Autodesk Inventor part; units mm, degrees
ref_plane "YZ Plane" through (0, 0, 0) normal (1, 0, 0) x (0, 1, 0)
ref_plane "XZ Plane" through (0, 0, 0) normal (0, 1, 0) x (-1, 0, 0)
ref_plane "XY Plane" through (0, 0, 0) normal (0, 0, 1) x (1, 0, 0)
sketch "スケッチ1" plane through (0, 0, 0) normal (1, 0, 0) x (0, 1, 0)
  line L0 (-54.6, 19) -> (54.6, 19)
  line L1 (58.6, 15) -> (58.6, -15)
  line L2 (54.6, -19) -> (-54.6, -19)
  line L3 (-58.6, -15) -> (-58.6, 15)
  line L4 (-58.6, 19) -> (58.6, -19) construction
  line L5 (58.6, 19) -> (-58.6, -19) construction
  arc A0 (-50.9799, 10.4) -> (-50.9799, 14.6) centre (-47, 12.5) ccw
  line L6 (-54.5, 10.4) -> (-50.9799, 10.4)
  line L7 (-54.5, 14.6) -> (-50.9799, 14.6)
  arc A1 (-54.5, 14.6) -> (-54.5, 10.4) centre (-54.5, 12.5) ccw
  line L8 (-54.5, 12.5) -> (-47, 12.5) construction
  line L9 (-58.6, 0) -> (58.6, 0) construction
  line L10 (-54.5, 19) -> (-54.5, -19) construction
  line L11 (-58.6, -19) -> (58.6, 19) construction
  line L12 (-54.5, -14.6) -> (-50.9799, -14.6)
  arc A2 (-54.5, -10.4) -> (-54.5, -14.6) centre (-54.5, -12.5) ccw
  line L13 (-54.5, -10.4) -> (-50.9799, -10.4)
  arc A3 (-50.9799, -14.6) -> (-50.9799, -10.4) centre (-47, -12.5) ccw
  line L14 (-54.5, -12.5) -> (-47, -12.5) construction
  line L15 (-54.5, -19) -> (-54.5, 19) construction
  line L16 (0, 19) -> (0, -19) construction
  line L17 (58.6, 19) -> (-58.6, -19) construction
  line L18 (-58.6, 19) -> (58.6, -19) construction
  line L19 (54.5, 14.6) -> (50.9799, 14.6)
  arc A4 (54.5, 10.4) -> (54.5, 14.6) centre (54.5, 12.5) ccw
  line L20 (54.5, 10.4) -> (50.9799, 10.4)
  arc A5 (50.9799, 14.6) -> (50.9799, 10.4) centre (47, 12.5) ccw
  line L21 (54.5, 12.5) -> (47, 12.5) construction
  line L22 (58.6, 0) -> (-58.6, 0) construction
  line L23 (54.5, 19) -> (54.5, -19) construction
  arc A6 (54.5, -14.6) -> (54.5, -10.4) centre (54.5, -12.5) ccw
  line L24 (54.5, -14.6) -> (50.9799, -14.6)
  line L25 (54.5, -10.4) -> (50.9799, -10.4)
  line L26 (54.5, -12.5) -> (47, -12.5) construction
  arc A7 (50.9799, -10.4) -> (50.9799, -14.6) centre (47, -12.5) ccw
  line L27 (54.5, -19) -> (54.5, 19) construction
  line L28 (58.6, -19) -> (-58.6, 19) construction
  arc A8 (-54.6, 19) -> (-58.6, 15) centre (-54.6, 15) ccw
  arc A9 (-58.6, -15) -> (-54.6, -19) centre (-54.6, -15) ccw
  arc A10 (58.6, 15) -> (54.6, 19) centre (54.6, 15) ccw
  arc A11 (54.6, -19) -> (58.6, -15) centre (54.6, -15) ccw
  line L29 (-20.5, 19) -> (-20.5, -19)
  line L30 (20.5, 19) -> (20.5, -19)
  line L31 (-16.5, 19) -> (-16.5, -19) construction
  line L32 (16.5, 19) -> (16.5, -19) construction
  line L33 (-24.5, 19) -> (-24.5, -19) construction
  line L34 (24.5, 19) -> (24.5, -19) construction
  circle A12 centre (-35.5, 12.5) radius 3.5
  circle A13 centre (-35.5, -12.5) radius 3.5
  circle A14 centre (35.5, 12.5) radius 3.5
  circle A15 centre (35.5, -12.5) radius 3.5
  point P0 (0, 0)
  point P1 (0, 0)
  point P2 (43.6458, 9.5001)
  point P3 (43.6458, 15.4999)
  point P4 (43.6458, -15.4999)
  point P5 (43.6458, -9.5001)
  point P6 (-43.6458, 15.4999)
  point P7 (-43.6458, 9.5001)
  point P8 (-43.6458, -9.5001)
  point P9 (-43.6458, -15.4999)
  dimension "d0" = 117.2
  dimension "d1" = 9
  dimension "d2" = 4.2
  dimension "d3" = 7.5
  dimension "d5" = 2
  dimension "d6" = 25
  dimension "d7" = 2
  dimension "d8" = 38
  dimension "d13" = 4
  dimension "d15" = 33
  dimension "d16" = 30
  dimension "d17" = 8
  dimension "d22" = 7
  dimension "d23" = 19
extrude "押し出し1" add sketch "スケッチ1" along normal blind 0.75
bend part "曲げパーツ1" radius 4 angle 90 line through (0, -20.5, 19) along (0, 0, -1) centre toward (-1, 0, 0) moving side (0, -1, 0) both sides no
bend part "曲げパーツ2" radius 4 angle 90 line through (0, 20.5, 19) along (0, 0, -1) centre toward (-1, 0, 0) moving side (0, 1, 0) both sides no
equation "\"d7\" = d5"
equation "\"d18\" = 0.5 * d17"
equation "\"d20\" = 0.5 * d17"
properties part number "Head_back_cloth"
Geometry: final body of the model. Coordinates: model frame, mm. A direction names the side the tool comes from. Coordinates: 2 decimals unless noted, no trailing zeros. Order: outer loops, then holes, each group sorted by start corner. A loop starts at its lowest first (then second) coordinate and runs counter-clockwise, first axis right, second up.
(1) Section query C-C (x = -2). Return the cut outline in (y, z), plus the area to 3 significant figures.
(2) Section query A-A (x = -14). Return the cut outline in (y, z).
(3) First-contact query: pin 1 (4 mm diameter, centred on x = -12.72, z = 12.5, fed in from +Y); pin 2 (1.5 mm diameter, centred on y = -8.5, z = 7.5, fed in from -X). Flat tips, straight axial feed; report the tip coordinate or a pass-through.
(4) Draft query along Y for faces 4 (the face through (-0.605, 23.822, 0.266)), 5 (the face through (-33.816, 24.87, 12.546)), 6 (the face through (0, 0, 0)). Return one class per face: pulls with the +Y half, pulls with the -Y half, needs draft (parallel to the pull), parting line crosses it, or undercut.
(5) Material intervals for probe 1 along Y at (x, z) = (-20, 2); probe 2 along X at (y, z) = (8, -7); probe 3 along X at (y, z) = (-24, 12), sorted ascending.
(6) Access query for faces 1 (the face through (-34.614, -24.87, -17.859)), 2 (the face through (-20, -24.5, 0)), 3 (the face through (-33.816, -24.87, 12.454)). Directions: +Z, -Z, +X, -X, +Y, -Y. A direction counts if a zero-diameter tool reaches every point of the face in a straight line with its end or side. Return the directions, or none.
(7) Section query D-D (y = -18.5). Return the cut outline in (x, z), plus the area to 3 significant figures.
(8) Section query B-B (z = -12.5). Return the cut outline in (x, y), plus the area to 3 significant figures.
Solution:
1. outline: (-24.81, -19) - (-23.96, -19) - (-23.96, 19) - (-24.81, 19) - close; (23.96, -19) - (24.81, -19) - (24.81, 19) - (23.96, 19) - close
1. area: 64.2 mm2
2. outline: (-25.25, -19) - (-24.5, -19) - (-24.5, -15.76) - (-25.25, -15.76) - close; (-25.25, -9.24) - (-24.5, -9.24) - (-24.5, 9.24) - (-25.25, 9.24) - close; (-25.25, 15.76) - (-24.5, 15.76) - (-24.5, 19) - (-25.25, 19) - close; (24.5, -19) - (25.25, -19) - (25.25, -15.76) - (24.5, -15.76) - close; (24.5, -9.24) - (25.25, -9.24) - (25.25, 9.24) - (24.5, 9.24) - close; (24.5, 15.76) - (25.25, 15.76) - (25.25, 19) - (24.5, 19) - close
3. pin 1: passes through
3. pin 2: stops at x = 0
4. face 4: pulls with the +Y half
4. face 5: needs draft
4. face 6: undercut
5. probe 1: y = -25.25 to -24.5, 24.5 to 25.25
5. probe 2: x = 0 to 0.75
5. probe 3: x = -2.06 to -0.79
6. face 1: -Z, -X, +Y, -Y
6. face 2: +Z, -Z, -X
6. face 3: +Y, -Y
7. outline: (0, -19) - (0.75, -19) - (0.75, 19) - (0, 19) - close
7. area: 28.5 mm2
8. outline: (-35.82, -25.25) - (-33.82, -25.25) - (-33.82, -24.5) - (-35.82, -24.5) - close; (-35.82, 24.5) - (-33.82, 24.5) - (-33.82, 25.25) - (-35.82, 25.25) - close; (-19.72, -25.25) - (-16.22, -25.25) - (-16.22, -24.5) - (-19.72, -24.5) - close; (-19.72, 24.5) - (-16.22, 24.5) - (-16.22, 25.25) - (-19.72, 25.25) - close; (-9.22, -25.25) - (-4, -25.25) arc R4.75 ccw to (0.75, -20.5) - (0.75, 20.5) arc R4.75 ccw to (-4, 25.25) - (-9.22, 25.25) - (-9.22, 24.5) - (-4, 24.5) arc R4 cw to (0, 20.5) - (0, -20.5) arc R4 cw to (-4, -24.5) - (-9.22, -24.5) - close
8. area: 57.1 mm2
